```python
from build123d import *

# Parameters (mm, degrees)
SKIZZE1_R                       = 15
AUFSATZ_LINEAR_AUSTRAGEN1_DEPTH = 3
VERRUNDUNG1_R                   = 16
VERRUNDUNG2_R                   = 5


# Read off the part's stored shape, not the designer's step: Wandung1
with BuildPart() as part:
    # Skizze2 → Rotation1 (revolve)
    with BuildSketch(Plane.XY, mode=Mode.PRIVATE) as rotation1_sk:
        Polygon((0, -134), (4.5, -134), (4.5, -126), (15, -124), (15, 0), (0, 0), align=None)
    revolve(rotation1_sk.sketch.rotate(Axis((0, 0, 0), (0, -1, 0)), 180), axis=Axis((0, 0, 0), (0, -1, 0)))

    # Wandung1 outline → Wandung1 (revolve, cut)
    with BuildSketch(Plane.XY):
        Polygon((0, -134), (3.75, -134), (3.75, -125.124878175), (14, -123.172497223), (14, 0), (0, 0), align=None)
    revolve(axis=Axis((0, 0, 0), (0, 1, 0)), mode=Mode.SUBTRACT)

    # Skizze1 → Aufsatz-Linear austragen1 (add)
    with BuildSketch(Plane(origin=(0, 0, 0), x_dir=(1, 0, 0), z_dir=(0, 1, 0))):
        Polygon((0, -19), (25.5, -10.5), (25.5, 10.5), (0, 19), (-25.5, 10.5), (-25.5, -10.5), align=None)
        with Locations(Location((0, 0, 0), (0, 0, 180))):
            Circle(SKIZZE1_R, mode=Mode.SUBTRACT)
    extrude(amount=-AUFSATZ_LINEAR_AUSTRAGEN1_DEPTH)

    # Verrundung1
    verrundung1_edges = [part.edges().sort_by_distance(p)[0] for p in [
        (0, -1.5, 19),
        (0, -1.5, -19),
    ]]
    fillet(verrundung1_edges, radius=VERRUNDUNG1_R)

    # Verrundung2
    verrundung2_edges = [part.edges().sort_by_distance(p)[0] for p in [
        (-25.5, -1.5, 10.5),
        (-25.5, -1.5, -10.5),
        (25.5, -1.5, -10.5),
        (25.5, -1.5, 10.5),
    ]]
    fillet(verrundung2_edges, radius=VERRUNDUNG2_R)


solid = part.part
```
Geometry check sheet. Reference: the model listing, model coordinates, mm. A direction names the side the tool comes from. Coordinates: 2 decimals unless noted, no trailing zeros. Order: outer loops, then holes, each group sorted by start corner. A loop starts at its lowest first (then second) coordinate and runs counter-clockwise, first axis right, second up. Notation, with made-up numbers: (47.5, 26) - (87.5, 26) arc R29 ccw to (87.5, 54) - close; hole circle Ø4 at (18.5, 62). An arc over 180 degrees is marked (long way). Use one line per item in the form item = value.
1. Access from +Z, -Z, +X, -X, +Y, -Y to the whole of each face (thin tool, end or side, straight path). Record for faces 4 (the face through (0, -3, 16)), 5 (the face through (12.932, -60.724, 5.362)), 6 (the face through (-12, 0, -8)).
Here are the results:
face_4 = -Y
face_5 = +Y
face_6 = +Z, -Z, +X, -X, +Y
2. Scan lines: line 1 (Z direction, x = 0, y = -47); line 2 (Z direction, x = 0, y = -128); line 3 (Y direction, x = -20, z = 2). Record each from-to range of solid material in increasing order.
Here are the results:
line_1 = -15 to -14, 14 to 15
line_2 = -4.5 to -3.75, 3.75 to 4.5
line_3 = -3 to 0
3. Draft check along Z on faces 1 (the face through (-3.746, -129.5, -0.165)), 2 (the face through (24.582, -1.521, -9.784)), 3 (the face through (-8.06, -62.65, -12.65)). Enter one of: pulls with the +Z half, pulls with the -Z half, needs draft (parallel to the pull), parting line crosses it, or undercut.
Here are the results:
face_1 = undercut
face_2 = pulls with the -Z half
face_3 = parting line crosses it
4. Section check C-C (y = -62). Record the boundary of the cut face in (x, z).
Here are the results:
outline = circle Ø30 at (0, 0); hole circle Ø28 at (0, 0)
5. Section check A-A (x = 0). Record the boundary of the cut face in (y, z), then the cut area to 3 significant figures.
Here are the results:
outline = (-134, -4.5) - (-126, -4.5) - (-124, -15) - (-3, -15) - (-3, -18.13) - (0, -18.13) - (0, -14) - (-123.17, -14) - (-125.12, -3.75) - (-134, -3.75) - close; (-134, 3.75) - (-125.12, 3.75) - (-123.17, 14) - (0, 14) - (0, 18.13) - (-3, 18.13) - (-3, 15) - (-124, 15) - (-126, 4.5) - (-134, 4.5) - close
area = 300 mm²
6. Section check B-B (z = 0). Record the boundary of the cut face in (x, y).
Here are the results:
outline = (-25.5, -3) - (-15, -3) - (-15, -124) - (-4.5, -126) - (-4.5, -134) - (-3.75, -134) - (-3.75, -125.12) - (-14, -123.17) - (-14, 0) - (-25.5, 0) - close; (3.75, -134) - (4.5, -134) - (4.5, -126) - (15, -124) - (15, -3) - (25.5, -3) - (25.5, 0) - (14, 0) - (14, -123.17) - (3.75, -125.12) - close
7. Gauge pin test, flat ends, axial feed: pin 1 (10 mm diameter, centred on y = -101.5, z = 5.5, fed in from +X); pin 2 (11 mm diameter, centred on x = -9.5, z = -5, fed in from -Y); pin 3 (4 mm diameter, centred on x = -10.5, y = -22.5, fed in from +Z). Record the tip position at first contact, or that the pin passes through.
Here are the results:
pin_1 = 14.99
pin_2 = -125.86
pin_3 = 12.36
